from build123d import *

# Parameters (mm, degrees)
CROQUIS1_R              = 1.125
SALIENTE_EXTRUIR1_DEPTH = 2
CROQUIS3_W              = 7
CROQUIS3_H              = 2.5
SALIENTE_EXTRUIR2_DEPTH = 2


with BuildPart() as part:
    # Croquis1 → Saliente-Extruir1 (new body)
    with BuildSketch(Plane(origin=(0, 0, 0), x_dir=(1, 0, 0), z_dir=(0, 1, 0))):
        with BuildLine():
            Line((19.91, 0), (11.125, 0))
            ThreePointArc((11.125, 0), (7.589466094, -1.464466094), (6.125, -5))
            ThreePointArc((6.125, -5), (0, -11.125), (-6.125, -5))
            ThreePointArc((-6.125, -5), (-7.589466094, -1.464466094), (-11.125, 0))
            Line((-11.125, 0), (-19.91, 0))
            ThreePointArc((-19.91, 0), (-22.031320344, 0.878679656), (-22.91, 3))
            Line((-22.91, 3), (-22.91, 10))
            Line((-22.91, 10), (-21.51, 10))
            Line((-21.51, 10), (-21.51, 12))
            Line((-21.51, 12), (-18.51, 12))
            Line((-18.51, 12), (-18.51, 10))
            Line((-18.51, 10), (-14.51, 10))
            Line((-14.51, 10), (-14.51, 12))
            Line((-14.51, 12), (-11.51, 12))
            Line((-11.51, 12), (-11.51, 10))
            Line((-11.51, 10), (-9.01, 10))
            ThreePointArc((-9.01, 10), (-6.888679656, 9.121320344), (-6.01, 7))
            Line((-6.01, 7), (-6.01, 1))
            Line((-6.01, 1), (6.01, 1))
            Line((6.01, 1), (6.01, 7))
            ThreePointArc((6.01, 7), (6.888679656, 9.121320344), (9.01, 10))
            Line((9.01, 10), (11.51, 10))
            Line((11.51, 10), (11.51, 12))
            Line((11.51, 12), (14.51, 12))
            Line((14.51, 12), (14.51, 10))
            Line((14.51, 10), (18.51, 10))
            Line((18.51, 10), (18.51, 12))
            Line((18.51, 12), (21.51, 12))
            Line((21.51, 12), (21.51, 10))
            Line((21.51, 10), (22.91, 10))
            Line((22.91, 10), (22.91, 3))
            ThreePointArc((22.91, 3), (22.031320344, 0.878679656), (19.91, 0))
        make_face()
        with Locations(Location((-16.51, 3, 0), (0, 0, 270))):
            Circle(CROQUIS1_R, mode=Mode.SUBTRACT)
        with Locations(Location((16.51, 3, 0), (0, 0, 90))):
            Circle(CROQUIS1_R, mode=Mode.SUBTRACT)
        with Locations(Location((0, -5, 0), (0, 0, 270))):
            Circle(CROQUIS1_R, mode=Mode.SUBTRACT)
    extrude(amount=SALIENTE_EXTRUIR1_DEPTH)

    # Croquis3 → Saliente-Extruir2 (add)
    with BuildSketch(Plane.XZ):
        with Locations((-16.51, -6.75)):
            Rectangle(CROQUIS3_W, CROQUIS3_H)
        with Locations((16.51, -6.75)):
            Rectangle(CROQUIS3_W, CROQUIS3_H)
    extrude(amount=SALIENTE_EXTRUIR2_DEPTH)


solid = part.part
Part model, mm, in its own coordinate system. A direction names the side the tool comes from. Give positions to 0.01 mm unless a question says otherwise; leave off trailing zeros. Order: outer loops, then holes, each group sorted by start corner. A loop starts at its lowest first (then second) coordinate and runs counter-clockwise, first axis right, second up. Notation, with made-up numbers: (51, 59.25) - (78, 59.25) arc R33 cw to (78, 98.25) - close; hole circle Ø3 at (-5.75, 39.25). An arc over 180 degrees is marked (long way). One line per question, with ' | ' between items.
1. Drill centre lines: probe 1 along X at (y, z) = (1.6, -3) (3 decimals); probe 2 along Z at (x, y) = (16.51, 0.65) (3 decimals); probe 3 along Y at (x, z) = (-1, 6.25). Where is each one in solid material? Low to high.
Filled in:
probe 1: -22.91 to -17.635, -15.385 to -6.01, 6.01 to 15.385, 17.635 to 22.91 | probe 2: -10 to -4.125, -1.875 to 0 | probe 3: 0 to 2
2. Drop flat-ended pins along their axis: P1, Ø1, axis at x = 16, y = 1, coming from the -Z side; P2, Ø1.6, axis at y = -1.5, z = -7.5, coming from the +X side; P3, Ø0.6, axis at y = -0.5, z = -6.5, coming from the -X side; P4, Ø2, axis at y = -1.5, z = 3, coming from the +X side. Give the stop position or say it passes through.
Filled in:
P1: z = -10 | P2: x = 20.01 | P3: x = -20.01 | P4: through
3. Band-saw the part on C-C on x = 0. List the corners of the cut face in (y, z) (3 decimals), then the cut area to 4 significant figures.
Filled in:
outline: (0, -1) - (2, -1) - (2, 3.875) - (0, 3.875) - close; (0, 6.125) - (2, 6.125) - (2, 11.125) - (0, 11.125) - close | area: 19.75 mm²
4. Pull direction Z, two halves, no side cores. Call faces 4 (the face through (-17, -1, -5.5)), 5 (the face through (-20, 1, -12)), 6 (the face through (-18.51, 1, -11)), 7 (the face through (0.049, 0.986, 3.876)): +Z half, -Z half, draft (parallel to the pull), parting line (faces both ways), or undercut.
Filled in:
face 4: +Z half | face 5: -Z half | face 6: draft | face 7: undercut
5. Band-saw the part on D-D on y = 1.5. Give the number of separate pieces and of enclosed holes in the cut face, then the cut area to 3 significant figures.
Filled in:
separate pieces: 1 | enclosed holes: 3 | area: 485 mm²
6. Band-saw the part on B-B on y = -1.4. List the corners of the cut face in (x, z), then the cut area to 3 significant figures.
Filled in:
outline: (-20.01, -8) - (-13.01, -8) - (-13.01, -5.5) - (-20.01, -5.5) - close; (13.01, -8) - (20.01, -8) - (20.01, -5.5) - (13.01, -5.5) - close | area: 35.0 mm²
7. Which spindle directions (+Z, -Z, +X, -X, +Y, -Y) get a long thin tool onto all of the face, cutting with end or side? Do faces 1 (the face through (-20.01, -1, -7)), 2 (the face through (16, 1, -10)), 3 (the face through (-13.01, -1, -7)). Say none if no direction does.
Filled in:
face 1: +Z, -Z, -X, -Y | face 2: -Z, +Y, -Y | face 3: +Z, -Z, -Y
8. Band-saw the part on A-A on x = 16.51. List the corners of the cut face in (y, z) (3 decimals).
Filled in:
outline: (-2, -8) - (0, -8) - (0, -10) - (2, -10) - (2, -4.125) - (0, -4.125) - (0, -5.5) - (-2, -5.5) - close; (0, -1.875) - (2, -1.875) - (2, 0) - (0, 0) - close
